```python
from build123d import *

# Parameters (mm, degrees)
CIRCLE001_R    = 8.697725
EXTRUDE_DEPTH  = 1
CYLINDER_R     = 5
CYLINDER_DEPTH = 15


with BuildPart() as obj1:
    # Circle001 → Extrude (new body)
    with BuildSketch(Plane.XY.offset(57.640399)):
        Circle(CIRCLE001_R)
    extrude(amount=EXTRUDE_DEPTH)


with BuildPart() as obj1_1:
    # Extrude placement: moved
    add(obj1.part.moved(Location((0, 0, -8.594981))))


with BuildPart() as obj2:
    # Cylinder → Cylinder (new body)
    with BuildSketch(Plane.XY.offset(42.640399)):
        Circle(CYLINDER_R)
    extrude(amount=CYLINDER_DEPTH)

    # Fusion002: union obj1
    add(obj1_1.part)


solid = obj2.part
```
Work out the finished part from the listing and answer in its coordinate system (mm). A direction names the side the tool comes from. Coordinates: 2 decimals unless noted, no trailing zeros. Loops run counter-clockwise (first coordinate to the right, second up) from the corner with the lowest first, then second, coordinate; pieces in that order, holes last.
1) For faces 1 (the cylindrical face through (8.3, 2.6, 49.5)), 2 (the cylindrical face through (-1.08, -4.88, 53.79)), 3 (the cylindrical face through (-1.08, -4.88, 45.8)), determine the directions among +Z, -Z, +X, -X, +Y, -Y from which every point of the face is accessible in a straight line to the end or side of a thin tool.
Results:
face 1: +Z, -Z
face 2: +Z
face 3: -Z
2) Consider probe 1 along Y at (x, z) = (0, 50.5); probe 2 along Z at (x, y) = (-2, -7.5). Determine where each line is inside the solid, lowest interval first.
Results:
probe 1: y = -5 to 5
probe 2: z = 49.05 to 50.05
3) Flat-ended cylindrical pins translate along their axes: pin 1 (3 mm diameter, centred on x = -1, z = 44, fed in from +Y); pin 2 (4 mm diameter, centred on y = 3.5, z = 56, fed in from +X); pin 3 (1 mm diameter, centred on x = -1, z = 52.5, fed in from -Y). Find the tip coordinate at first contact, or state that the pin passes through.
Results:
pin 1: stops at y = 5
pin 2: stops at x = 4.77
pin 3: stops at y = -4.97
4) Section A-A (y = 0) is taken. Give the vertices of the cut face in (x, z), plus the area to 3 significant figures.
Results:
outline: (-8.7, 49.05) - (-5, 49.05) - (-5, 42.64) - (5, 42.64) - (5, 49.05) - (8.7, 49.05) - (8.7, 50.05) - (5, 50.05) - (5, 57.64) - (-5, 57.64) - (-5, 50.05) - (-8.7, 50.05) - close
area: 157 mm2
5) Section D-D (x = -7.5) is taken. Give the vertices of the cut face in (y, z).
Results:
outline: (-4.4, 49.05) - (4.4, 49.05) - (4.4, 50.05) - (-4.4, 50.05) - close
6) Section C-C (z = 45.5) is taken. Give the vertices of the cut face in (x, y).
Results:
outline: circle Ø10 at (0, 0)
